from build123d import *

# Parameters (mm, degrees)
F1_DEPTH = 25
F2_T     = -2
F4_DEPTH = 25


with BuildPart() as f1:
    # F0 (on Front) → F1 (new body, symmetric)
    with BuildSketch(Plane.XZ):
        with BuildLine():
            Line((50, 10), (-50, 10))
            Line((-50, 10), (-50, -5))
            ThreePointArc((-50, -5), (-48.5355339059, -8.5355339059), (-45, -10))
            Line((-45, -10), (45, -10))
            ThreePointArc((45, -10), (48.5355339059, -8.5355339059), (50, -5))
            Line((50, -5), (50, 10))
        make_face()
    extrude(amount=F1_DEPTH, both=True)

    # F2
    f2_openings = [f1.faces().sort_by_distance(p)[0] for p in [
        (0, 0, 10),
    ]]
    offset(amount=F2_T, openings=f2_openings)

    # F3 (on face) → F4 (join)
    with BuildSketch(Plane.XY.offset(10)):
        with BuildLine():
            Line((48, -18.7663880923), (48, -21.7598285526))
            Line((48, -21.7598285526), (48, -23))
            Line((48, -23), (46.7598285526, -23))
            Line((46.7598285526, -23), (43.7663880923, -23))
            ThreePointArc((43.7663880923, -23), (44.9597809557, -24.4539962641), (46.7598286169, -25))
            ThreePointArc((46.7598286169, -25), (49.050975778, -24.0509757325), (50, -21.7598285526))
            ThreePointArc((50, -21.7598285526), (49.4539962462, -19.959780929), (48, -18.7663880923))
        make_face()
        with BuildLine():
            ThreePointArc((46.7598285526, -23), (45.8828949123, -20.8828949123), (48, -21.7598285526))
            Line((48, -21.7598285526), (48, -18.7663880923))
            ThreePointArc((48, -18.7663880923), (44.4686813499, -19.4686813499), (43.7663880923, -23))
            Line((43.7663880923, -23), (46.7598285526, -23))
        make_face()
    extrude(amount=-F4_DEPTH)


solid = f1.part
Can you work these out from the model? Positions are in its coordinate system, mm. A direction names the side the tool comes from. Coordinates: 2 decimals unless noted, no trailing zeros. Write each loop counter-clockwise with the first axis right and the second up, starting at its lowest first coordinate (ties: lowest second). Pieces come first, ordered by that corner, then holes. Notation, with made-up numbers: (87.25, 75.5) -> (139.25, 75.5) arc R35 cw to (139.25, 113.5) -> close; hole circle Ø11 at (64, 29.25). An arc over 180 degrees is marked (long way). Write each question's results on one line, items separated by ' | '. Start each with the question number.
Item 1: If we section it at A-A, the plane z = 0.75: Write out the boundary of the cut face in (x, y), and give its area (3 significant figures).
Item 2: If we section it at C-C, the plane x = 38.5: Write out the boundary of the cut face in (y, z), and give its area (3 significant figures).
Item 3: If we section it at B-B, the plane y = 13: Write out the boundary of the cut face in (x, z).
Item 4: On a 3-axis mill with a long thin cutter (end or side, diameter ignored), from which of +Z, -Z, +X, -X, +Y, -Y can I reach the whole of each face in a straight line? I mean faces 1 (the flat face through (-48, 0, 3)), 2 (the cylindrical face through (45.854, -20.912, -11.958)), 3 (the cylindrical face through (-49, 0, -8)). Say none if no direction works.
Item 5: Please list where these lines run through material, in increasing order: probe 1 along Y at (x, z) = (-9.5, 4); probe 2 along X at (y, z) = (11.5, -1.5); probe 3 along Z at (x, y) = (-31.5, 9.5).
Item 6: Thinking about a two-plate mould opening in X: for faces 4 (the flat face through (-1, 25, 0)), 5 (the cylindrical face through (49.706, -24.123, -6.691)), 6 (the cylindrical face through (45.854, -20.912, 1.148)), which applies, released by +X, released by -X, zero draft, split by the parting line, or undercut?
Item 7: I'm going to push flat-ended pins straight in: P1, Ø2, axis at x = 46.76, y = -21.76, coming from the -Z side; P2, Ø3, axis at x = 46.76, y = -21.76, coming from the -Z side; P3, Ø1, axis at x = -2, y = -1, coming from the +Z side; P4, Ø25, axis at x = 17.5, y = 1.5, coming from the -Z side. Where does each tip first touch, or does it pass through?
Answer block:
1) outline: (-50, -25) -> (50, -25) -> (50, 25) -> (-50, 25) -> close; hole (-48, -23) -> (43.77, -23) arc R3.24 cw to (48, -18.77) -> (48, 23) -> (-48, 23) -> close; hole (46.76, -23) -> (48, -23) -> (48, -21.76) arc R1.24 ccw (long way) to start | area: 596 mm²
2) outline: (-25, -10) -> (25, -10) -> (25, 10) -> (23, 10) -> (23, -8) -> (-23, -8) -> (-23, 10) -> (-25, 10) -> close | area: 172 mm²
3) outline: (-50, -5) arc R5 ccw to (-45, -10) -> (45, -10) arc R5 ccw to (50, -5) -> (50, 10) -> (48, 10) -> (48, -5) arc R3 cw to (45, -8) -> (-45, -8) arc R3 cw to (-48, -5) -> (-48, 10) -> (-50, 10) -> close
4) face 1: +Z | face 2: -Z | face 3: -Z, -X, +Y, -Y
5) probe 1: -25 to -23, 23 to 25 | probe 2: -50 to -48, 48 to 50 | probe 3: -10 to -8
6) face 4: zero draft | face 5: released by +X | face 6: undercut
7) P1: z = -9.94 | P2: z = -15 | P3: z = -8 | P4: z = -10
